```python
from build123d import *

# Parameters (mm, degrees)
D_ME1_FACE_RADIUS = 2
D_ME1_HEIGHT      = 1


with BuildPart() as part:
    # Esquisse1 → Révolution1 (revolve)
    with BuildSketch(Plane.XY):
        Polygon((0, 0), (0, 2), (8, 2), (8, 3), (9.4, 3), (9.4, 2), (14.4, 2), (14.4, 0), align=None)
    revolve(axis=Axis((14.4, 0, 0), (-1, 0, 0)))

    # Dôme1: a dome of height H over a round flat face of radius A is a cap of a sphere of radius (A * A + H * H) / (2 * H)
    d_me1_r = (D_ME1_FACE_RADIUS * D_ME1_FACE_RADIUS + D_ME1_HEIGHT * D_ME1_HEIGHT) / (2 * D_ME1_HEIGHT)
    d_me1_base = Plane((14.4, 0, 0), z_dir=(1, 0, 0))
    with Locations(d_me1_base.offset(D_ME1_HEIGHT - d_me1_r)):
        d_me1_ball = Sphere(d_me1_r, mode=Mode.PRIVATE)
    add(split(d_me1_ball, bisect_by=d_me1_base, keep=Keep.TOP, mode=Mode.PRIVATE))


solid = part.part
```
Design review of the part built by this model. Coordinates are the model's own, in mm. A direction names the side the tool comes from. Round coordinates to 2 decimals unless told otherwise and drop trailing zeros. Write each loop counter-clockwise with the first axis right and the second up, starting at its lowest first coordinate (ties: lowest second). Pieces come first, ordered by that corner, then holes. Notation, with made-up numbers: (51.25, 2) -> (73.25, 2) arc R34 ccw to (73.25, 35) -> close; hole circle Ø2 at (-3, -28.75). An arc over 180 degrees is marked (long way). Answer in a Markdown table with one row per item.
Q1. Take a section at D-D, the plane x = 8.75. State the section outline as (y, z) points.
The answers:
| item | result |
|---|---|
| outline | circle Ø6 at (0, 0) |
Q2. For faces 1 (the face through (4, 0, 2)), 2 (the face through (0, 0, 0)), 3 (the face through (12, 0, 2)), list the 3-axis set-ups (+Z, -Z, +X, -X, +Y, -Y) from which the entire face can be reached by the end or side of a thin tool; tool diameter is ignored.
The answers:
| item | result |
|---|---|
| face 1 | -X |
| face 2 | +Z, -Z, -X, +Y, -Y |
| face 3 | +X |
Q3. Clearance check with flat-ended pins moving along their axes: pin 1 Ø2 at (x, y) = (4.5, -1) entering from +Z; pin 2 Ø3 at (y, z) = (1.5, 1.5) entering from +X. State where each tip first meets the part, or that it passes through.
The answers:
| item | result |
|---|---|
| pin 1 | z = 2 |
| pin 2 | x = 15.32 |
Q4. Take a section at C-C, the plane x = 4.5. State the section outline as (y, z) points.
The answers:
| item | result |
|---|---|
| outline | circle Ø4 at (0, 0) |
Q5. To check wall thickness, follow L1, parallel to Y at x = 1, z = 0.1; L2, parallel to X at y = -0.95, z = 2.7. State the ranges of each line that lie inside material, in increasing order. Write a range as [from, to].
The answers:
| item | result |
|---|---|
| L1 | [-2, 2] |
| L2 | [8, 9.4] |
Q6. Take a section at A-A, the plane z = 0. State the section outline as (x, y) points, then the cut area to 3 significant figures.
The answers:
| item | result |
|---|---|
| outline | (0, -2) -> (8, -2) -> (8, -3) -> (9.4, -3) -> (9.4, -2) -> (14.4, -2) arc R2.5 ccw to (14.4, 2) -> (9.4, 2) -> (9.4, 3) -> (8, 3) -> (8, 2) -> (0, 2) -> close |
| area | 63.2 mm² |
